Read the model definition and answer for the solid it produces. Units are mm, in the model's axes. Face numbers are marked on the shaded views. Coordinates: 2 decimals unless noted, no trailing zeros. Write each loop counter-clockwise with the first axis right and the second up, starting at its lowest first coordinate (ties: lowest second). Pieces come first, ordered by that corner, then holes.
Item 1: Section B-B (x = 0) is taken. Give the vertices of the cut face in (y, z), then the cut area to 3 significant figures.
Item 2: Each of these flat-tipped pins is pushed along its axis until it touches: P1, Ø3, axis at x = -81.5, y = -2, coming from the +Z side; P2, Ø10, axis at x = -63, y = 19, coming from the +Z side; P3, Ø0.9, axis at y = 20, z = 28.5, coming from the +X side. Where does it stop, or does it pass through?
Item 3: Section D-D (x = -48) is taken. Give the vertices of the cut face in (y, z) (3 decimals), then the cut area to 3 significant figures.
Item 4: Section C-C (y = 14.25) is taken. Give the vertices of the cut face in (x, z), then the cut area to 3 significant figures.
Item 5: Straight lines are drawn through the part: probe 1 along Z at (x, y) = (-65, 6); probe 2 along X at (y, z) = (3.25, -10.5); probe 3 along X at (y, z) = (11.75, 0.5). For each, find the intervals that lie inside material, in ascending order.
Item 6: Determine the mould class of the marked faces 1, 2, 3 and 4 for opening direction X: released by +X, released by -X, zero draft, split by the parting line, or undercut.
Item 7: Section A-A (z = 0) is taken. Give the vertices of the cut face in (x, y), then the cut area to 3 significant figures.
from build123d import *

# Parameters (mm, degrees)
SKETCH1_R            = 44.45
BOSS_EXTRUDE1_DEPTH  = 19.05
BOSS_EXTRUDE2_DEPTH  = 3.175
SKETCH4_W            = 53.981480267
SKETCH4_H            = 15.875
BOSS_EXTRUDE3_DEPTH  = 7.62
SKETCH5_W            = 53.981480267
SKETCH5_H            = 15.875
BOSS_EXTRUDE4_DEPTH  = 7.62
SKETCH2_R            = 38.1
CUT_EXTRUDE1_DEPTH   = 98.872432789
CUT_EXTRUDE1_DRAFT   = 14
SKETCH6_W            = 6.35
SKETCH6_H            = 2.9972
BOSS_EXTRUDE5_DEPTH  = 3.429
FILLET1_R            = 0.508
FILLET1_OF_MIRROR1_R = 0.508


with BuildPart() as part:
    # Sketch1 → Boss-Extrude1 (new body)
    with BuildSketch(Plane(origin=(0, 0, 0), x_dir=(1, 0, 0), z_dir=(0, 1, 0))):
        with Locations(Location((0, 0, 0), (0, 0, 90))):
            Circle(SKETCH1_R)
    extrude(amount=BOSS_EXTRUDE1_DEPTH)

    # Sketch3 → Boss-Extrude2 (add)
    with BuildSketch(Plane.XZ):
        with BuildLine():
            Line((-31.108519733, 31.75), (-85.09, 31.75))
            Line((-85.09, 31.75), (-85.09, 6.35))
            Line((-85.09, 6.35), (-43.994090512, 6.35))
            ThreePointArc((-43.994090512, 6.35), (-39.640768363, 20.109997105), (-31.108519733, 31.75))
        make_face()
    extrude(amount=-BOSS_EXTRUDE2_DEPTH)

    # Sketch4 → Boss-Extrude3 (add)
    with BuildSketch(Plane.XY.offset(31.75)):
        with Locations((-58.099259867, 11.1125)):
            Rectangle(SKETCH4_W, SKETCH4_H)
    extrude(amount=-BOSS_EXTRUDE3_DEPTH)

    # Sketch5 → Boss-Extrude4 (add)
    with BuildSketch(Plane(origin=(0, 0, 6.35), x_dir=(-1, 0, 0), z_dir=(0, 0, -1))):
        with Locations((58.099259867, 11.1125)):
            Rectangle(SKETCH5_W, SKETCH5_H)
    extrude(amount=-BOSS_EXTRUDE4_DEPTH)


with BuildPart() as cut_extrude1_tool:
    # Sketch2 → Cut-Extrude1 (with draft: the straight prism first)
    with BuildSketch(Plane.XZ):
        Circle(SKETCH2_R)
    extrude(amount=-CUT_EXTRUDE1_DEPTH)
    # Cut-Extrude1: the draft: its side faces are tilted about the plane it starts from
    cut_extrude1_sides = [cut_extrude1_tool.faces().sort_by_distance(p)[0] for p in [
        (-38.1, 49.436216394, 0),
    ]]
    draft(cut_extrude1_sides, Plane.XZ, CUT_EXTRUDE1_DRAFT)


with BuildPart() as part_1:
    add(part.part)

    # Cut-Extrude1: cut by cut_extrude1_tool
    add(cut_extrude1_tool.part, mode=Mode.SUBTRACT)

    # Sketch6 → Boss-Extrude5 (add)
    with BuildSketch(Plane(origin=(0, 19.05, 0), x_dir=(1, 0, 0), z_dir=(0, 1, 0))):
        with Locations((-81.915, -27.94)):
            Rectangle(SKETCH6_W, SKETCH6_H)
        with Locations((-69.215, -27.94)):
            Rectangle(SKETCH6_W, SKETCH6_H)
        with Locations((-56.515, -27.94)):
            Rectangle(SKETCH6_W, SKETCH6_H)
        with Locations((-56.515, -10.16)):
            Rectangle(SKETCH6_W, SKETCH6_H)
        with Locations((-69.215, -10.16)):
            Rectangle(SKETCH6_W, SKETCH6_H)
        with Locations((-81.915, -10.16)):
            Rectangle(SKETCH6_W, SKETCH6_H)
    boss_extrude5 = extrude(amount=BOSS_EXTRUDE5_DEPTH)

    # Fillet1
    fillet1_edges = [part_1.edges().sort_by_distance(p)[0] for p in [
        (-69.215, 22.479, 29.4386),
        (-66.04, 22.479, 27.94),
        (-69.215, 22.479, 26.4414),
        (-72.39, 22.479, 27.94),
        (-85.09, 22.479, 27.94),
        (-81.915, 22.479, 29.4386),
        (-78.74, 22.479, 27.94),
        (-81.915, 22.479, 26.4414),
        (-85.09, 22.479, 10.16),
        (-81.915, 22.479, 11.6586),
        (-78.74, 22.479, 10.16),
        (-81.915, 22.479, 8.6614),
        (-72.39, 22.479, 10.16),
        (-69.215, 22.479, 11.6586),
        (-66.04, 22.479, 10.16),
        (-69.215, 22.479, 8.6614),
        (-59.69, 22.479, 10.16),
        (-56.515, 22.479, 11.6586),
        (-53.34, 22.479, 10.16),
        (-56.515, 22.479, 8.6614),
        (-56.515, 22.479, 29.4386),
        (-53.34, 22.479, 27.94),
        (-56.515, 22.479, 26.4414),
        (-59.69, 22.479, 27.94),
    ]]
    fillet(fillet1_edges, radius=FILLET1_R)

    # Mirror1: Boss-Extrude5 across plane
    add(boss_extrude5.mirror(Plane.ZX.offset(9.525)))

    # Fillet1 of Mirror1
    fillet1_of_mirror1_edges = [part_1.edges().sort_by_distance(p)[0] for p in [
        (-69.215, -3.429, 29.4386),
        (-66.04, -3.429, 27.94),
        (-69.215, -3.429, 26.4414),
        (-72.39, -3.429, 27.94),
        (-85.09, -3.429, 27.94),
        (-81.915, -3.429, 29.4386),
        (-78.74, -3.429, 27.94),
        (-81.915, -3.429, 26.4414),
        (-85.09, -3.429, 10.16),
        (-81.915, -3.429, 11.6586),
        (-78.74, -3.429, 10.16),
        (-81.915, -3.429, 8.6614),
        (-72.39, -3.429, 10.16),
        (-69.215, -3.429, 11.6586),
        (-66.04, -3.429, 10.16),
        (-69.215, -3.429, 8.6614),
        (-59.69, -3.429, 10.16),
        (-56.515, -3.429, 11.6586),
        (-53.34, -3.429, 10.16),
        (-56.515, -3.429, 8.6614),
        (-56.515, -3.429, 29.4386),
        (-53.34, -3.429, 27.94),
        (-56.515, -3.429, 26.4414),
        (-59.69, -3.429, 27.94),
    ]]
    fillet(fillet1_of_mirror1_edges, radius=FILLET1_OF_MIRROR1_R)


solid = part_1.part
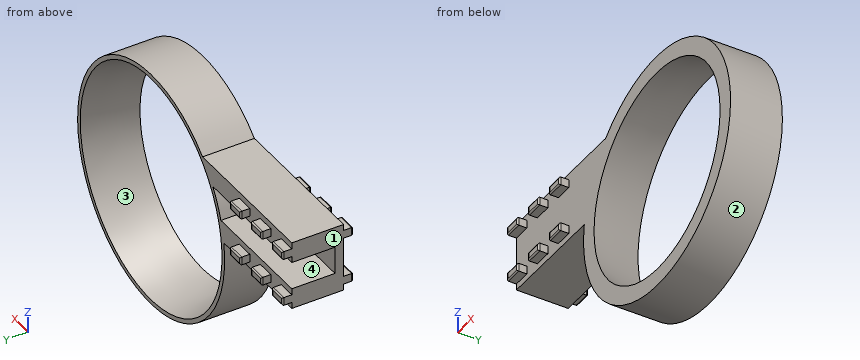
Established:
1. outline: (0, -44.45) - (19.05, -44.45) - (19.05, -42.85) - (0, -38.1) - close; (0, 38.1) - (19.05, 42.85) - (19.05, 44.45) - (0, 44.45) - close
1. area: 151 mm2
2. P1: stops at z = 29.44
2. P2: stops at z = 31.75
2. P3: stops at x = -53.34
3. outline: (0, 6.35) - (19.05, 6.35) - (19.05, 13.97) - (3.175, 13.97) - (3.175, 24.13) - (19.05, 24.13) - (19.05, 31.75) - (0, 31.75) - close
3. area: 323 mm2
4. outline: (-85.09, 6.35) - (-43.99, 6.35) arc R44.45 ccw (long way) to (-31.11, 31.75) - (-85.09, 31.75) - (-85.09, 24.13) - (-37.33, 24.13) arc R44.45 ccw to (-42.2, 13.97) - (-85.09, 13.97) - close; hole circle Ø83.31 at (0, 0)
4. area: 1,460 mm2
5. probe 1: z = 6.35 to 13.97, 24.13 to 31.75
5. probe 2: x = -43.19 to -37.47, 37.47 to 43.19
5. probe 3: x = -44.45 to -41.03, 41.03 to 44.45
6. face 1: released by -X
6. face 2: split by the parting line
6. face 3: undercut
6. face 4: zero draft
7. outline: (-44.45, 0) - (-38.1, 0) - (-42.85, 19.05) - (-44.45, 19.05) - close; (38.1, 0) - (44.45, 0) - (44.45, 19.05) - (42.85, 19.05) - close
7. area: 151 mm2
